Here's how the part is built. I have some questions about the finished solid (model axes, mm). A direction names the side the tool comes from. Coordinates: 2 decimals unless noted, no trailing zeros. Write each loop counter-clockwise with the first axis right and the second up, starting at its lowest first coordinate (ties: lowest second). Pieces come first, ordered by that corner, then holes.
```python
from build123d import *

# Parameters (mm, degrees)
EXTRUDE_1_DEPTH = 72
SKETCH_2_W      = 4
SKETCH_2_H      = 72
EXTRUDE_2_DEPTH = 3
SKETCH_4_W      = 60
SKETCH_4_H      = 11
EXTRUDE_3_DEPTH = 5


with BuildPart() as part:
    # 스케치1 → 보스-돌출1 (new body)
    with BuildSketch(Plane.XY):
        Polygon((-3, 0), (0, 0), (0, 4), (54, 4), (54, 0), (57, 0), (57, 8), (-3, 8), align=None)
    extrude(amount=EXTRUDE_1_DEPTH)

    # 스케치2 → 보스-돌출2 (add)
    with BuildSketch(Plane.XZ):
        with Locations((-1, 36)):
            Rectangle(SKETCH_2_W, SKETCH_2_H)
        with Locations((55, 36)):
            Rectangle(SKETCH_2_W, SKETCH_2_H)
    extrude(amount=EXTRUDE_2_DEPTH)

    # 스케치4 → 보스-돌출3 (add)
    with BuildSketch(Plane(origin=(0, 0, 0), x_dir=(-1, 0, 0), z_dir=(0, 0, -1))):
        with Locations((-27, 2.5)):
            Rectangle(SKETCH_4_W, SKETCH_4_H)
    extrude(amount=EXTRUDE_3_DEPTH)


solid = part.part
```
1) Will these pins go through, and if not, where does the flat tip stop? pin 1 (1 mm diameter, centred on x = 49.5, z = 14.5, fed in from -Y); pin 2 (3.5 mm diameter, centred on x = 20.5, y = -1, fed in from +Z).
Values follow:
pin 1: stops at y = 4
pin 2: stops at z = 0
2) Imagine slicing it at A-A on y = 3. Please give me the cut outline in (x, z), then the cut area to 3 significant figures.
Values follow:
outline: (-3, -5) - (57, -5) - (57, 72) - (54, 72) - (54, 0) - (0, 0) - (0, 72) - (-3, 72) - close
area: 732 mm2
3) On a 3-axis mill with a long thin cutter (end or side, diameter ignored), from which of +Z, -Z, +X, -X, +Y, -Y can I reach the whole of each face in a straight line? I mean faces 4 (the face through (53, -1, 35)), 5 (the face through (0, 2, 35)), 6 (the face through (27, 8, 34)). Say none if no direction works.
Values follow:
face 4: +Z, -Y
face 5: +Z
face 6: +Z, -Z, +X, -X, +Y
4) We'd pull the mould along X, two halves only. Please class faces 1 (the face through (54, 2, 35)), 2 (the face through (57, 2, 34)), 3 (the face through (-3, 2, 34)): pulls with the +X half, pulls with the -X half, needs draft (parallel to the pull), parting line crosses it, or undercut.
Values follow:
face 1: undercut
face 2: pulls with the +X half
face 3: pulls with the -X half
5) Imagine slicing it at D-D on y = -1. Please give me the cut outline in (x, z), then the cut area to 3 significant figures.
Values follow:
outline: (-3, -5) - (57, -5) - (57, 72) - (53, 72) - (53, 0) - (1, 0) - (1, 72) - (-3, 72) - close
area: 876 mm2
6) I need wall thicknesses on probe 1 along X at (y, z) = (1, 29); probe 2 along X at (y, z) = (-0.25, 52.5); probe 3 along Z at (x, y) = (36.5, -1.75). Which ranges of each line are inside material? Lowest first, please.
Values follow:
probe 1: x = -3 to 0, 54 to 57
probe 2: x = -3 to 1, 53 to 57
probe 3: z = -5 to 0
7) Imagine slicing it at B-B on z = 48.5. Please give me the cut outline in (x, y).
Values follow:
outline: (-3, -3) - (1, -3) - (1, 0) - (0, 0) - (0, 4) - (54, 4) - (54, 0) - (53, 0) - (53, -3) - (57, -3) - (57, 8) - (-3, 8) - close
8) Imagine slicing it at C-C on x = 7.5. Please give me the cut outline in (y, z).
Values follow:
outline: (-3, -5) - (8, -5) - (8, 72) - (4, 72) - (4, 0) - (-3, 0) - close
